from build123d import *
from build123d.topology import SkipClean

# Parameters (mm, degrees)
BOSS_EXTRUDE1_DEPTH       = 4
BOSS_EXTRUDE2_DEPTH       = 1
BOSS_EXTRUDE3_START       = -0.8
SKETCH4_R                 = 2
SKETCH4_R_2               = 1.25
BOSS_EXTRUDE3_DEPTH       = 3.2
MIRROR4_START             = -0.8
MIRROR4_COPY_1_SKETCH_R   = 2
MIRROR4_COPY_1_SKETCH_R_2 = 1.25
MIRROR4_COPY_1_DEPTH      = 3.2
SKETCH5_R                 = 4.5
CUT_EXTRUDE1_DEPTH        = 3
SKETCH1_R                 = 1.25
CUT_EXTRUDE2_DEPTH        = 10
FILLET2_R                 = 1
EXTRUDE_THIN1_START       = -4.2
SKETCH6_R                 = 2
SKETCH6_R_2               = 1
EXTRUDE_THIN1_DEPTH       = 4.2


with BuildPart() as part:
    # Sketch2 → Boss-Extrude1 (new body)
    with BuildSketch(Plane(origin=(0, 0, 0), x_dir=(1, 0, 0), z_dir=(0, 1, 0))):
        with BuildLine():
            Line((-26.6, 15.24), (-26.6, 2.54))
            ThreePointArc((-26.6, 2.54), (-25.504579362, -0.104579362), (-22.86, -1.2))
            Line((-22.86, -1.2), (-2.54, -1.2))
            ThreePointArc((-2.54, -1.2), (0.104579362, -0.104579362), (1.2, 2.54))
            Line((1.2, 2.54), (1.2, 15.24))
            ThreePointArc((1.2, 15.24), (0.104579362, 17.884579362), (-2.54, 18.98))
            Line((-2.54, 18.98), (-22.86, 18.98))
            ThreePointArc((-22.86, 18.98), (-25.504579362, 17.884579362), (-26.6, 15.24))
        make_face()
        with BuildLine():
            Line((0.2, 2.54), (0.2, 15.24))
            ThreePointArc((0.2, 15.24), (-0.60252742, 17.17747258), (-2.54, 17.98))
            Line((-2.54, 17.98), (-22.86, 17.98))
            ThreePointArc((-22.86, 17.98), (-24.79747258, 17.17747258), (-25.6, 15.24))
            Line((-25.6, 15.24), (-25.6, 2.54))
            ThreePointArc((-25.6, 2.54), (-24.79747258, 0.60252742), (-22.86, -0.2))
            Line((-22.86, -0.2), (-2.54, -0.2))
            ThreePointArc((-2.54, -0.2), (-0.60252742, 0.60252742), (0.2, 2.54))
        make_face(mode=Mode.SUBTRACT)
    extrude(amount=BOSS_EXTRUDE1_DEPTH)

    # Sketch3 → Boss-Extrude2 (add)
    with BuildSketch(Plane(origin=(0, 4, 0), x_dir=(1, 0, 0), z_dir=(0, 1, 0))):
        with BuildLine():
            Line((-26.6, 15.24), (-26.6, 2.54))
            ThreePointArc((-26.6, 2.54), (-25.504579362, -0.104579362), (-22.86, -1.2))
            Line((-22.86, -1.2), (-2.54, -1.2))
            ThreePointArc((-2.54, -1.2), (0.104579362, -0.104579362), (1.2, 2.54))
            Line((1.2, 2.54), (1.2, 15.24))
            ThreePointArc((1.2, 15.24), (0.104579362, 17.884579362), (-2.54, 18.98))
            Line((-2.54, 18.98), (-22.86, 18.98))
            ThreePointArc((-22.86, 18.98), (-25.504579362, 17.884579362), (-26.6, 15.24))
        make_face()
    extrude(amount=BOSS_EXTRUDE2_DEPTH)

    # Sketch4 → Boss-Extrude3 (add)
    # profile 1 of 2: a face of its own
    with BuildSketch(Plane.XZ.offset(BOSS_EXTRUDE3_START)):
        with BuildLine():
            ThreePointArc((-22.86, -4.54), (-24.274213562, -1.125786438), (-20.86, -2.54))
            Line((-20.86, -2.54), (-20.86, 0.2))
            Line((-20.86, 0.2), (-22.86, 0.2))
            ThreePointArc((-22.86, 0.2), (-24.79747258, -0.60252742), (-25.6, -2.54))
            Line((-25.6, -2.54), (-25.6, -4.54))
            Line((-25.6, -4.54), (-22.86, -4.54))
        make_face()
    # profile 2 of 2: a face of its own
    with BuildSketch(Plane.XZ.offset(BOSS_EXTRUDE3_START)):
        with Locations((-22.86, -2.54)):
            Circle(SKETCH4_R)
        with Locations(Location((-22.86, -2.54, 0), (0, 0, 90))):
            Circle(SKETCH4_R_2, mode=Mode.SUBTRACT)
    boss_extrude3 = extrude(amount=-BOSS_EXTRUDE3_DEPTH)

    # Mirror3: Boss-Extrude3 across plane
    add(boss_extrude3.mirror(Plane.ZY.offset(12.7)))

    # Mirror4: Boss-Extrude3 across plane
    add(boss_extrude3.mirror(Plane(origin=(0, 0, -8.89), x_dir=(1, 0, 0), z_dir=(0, 0, -1))))

    # Mirror4 copy 1 sketch → Mirror4 copy 1 (add)
    # profile 1 of 2: a face of its own
    with BuildSketch(Plane(origin=(-25.4, 0, -17.78), x_dir=(-1, 0, 0), z_dir=(0, -1, 0)).offset(MIRROR4_START)):
        with BuildLine():
            ThreePointArc((-22.86, -4.54), (-24.274213562, -1.125786438), (-20.86, -2.54))
            Line((-20.86, -2.54), (-20.86, 0.2))
            Line((-20.86, 0.2), (-22.86, 0.2))
            ThreePointArc((-22.86, 0.2), (-24.79747258, -0.60252742), (-25.6, -2.54))
            Line((-25.6, -2.54), (-25.6, -4.54))
            Line((-25.6, -4.54), (-22.86, -4.54))
        make_face()
    # profile 2 of 2: a face of its own
    with BuildSketch(Plane(origin=(-25.4, 0, -17.78), x_dir=(-1, 0, 0), z_dir=(0, -1, 0)).offset(MIRROR4_START)):
        with Locations((-22.86, -2.54)):
            Circle(MIRROR4_COPY_1_SKETCH_R)
        with Locations(Location((-22.86, -2.54, 0), (0, 0, 90))):
            Circle(MIRROR4_COPY_1_SKETCH_R_2, mode=Mode.SUBTRACT)
    extrude(amount=-MIRROR4_COPY_1_DEPTH)

    # Sketch5 → Cut-Extrude1 (cut)
    with BuildSketch(Plane(origin=(0, 5, 0), x_dir=(1, 0, 0), z_dir=(0, 1, 0))):
        with Locations(Location((-12.7, 8.89, 0), (0, 0, 270))):
            Circle(SKETCH5_R)
    extrude(amount=-CUT_EXTRUDE1_DEPTH, mode=Mode.SUBTRACT)

    # Sketch1 → Cut-Extrude2 (cut)
    with SkipClean():  # the faces are left unmerged after this step: merging them gives an invalid solid
        with BuildSketch(Plane(origin=(0, 0, 0), x_dir=(1, 0, 0), z_dir=(0, 1, 0))):
            with Locations(Location((-22.86, 2.54, 0), (0, 0, 270))):
                Circle(SKETCH1_R)
            with Locations(Location((-2.54, 2.54, 0), (0, 0, 270))):
                Circle(SKETCH1_R)
            with Locations(Location((-2.54, 15.24, 0), (0, 0, 270))):
                Circle(SKETCH1_R)
            with Locations(Location((-22.86, 15.24, 0), (0, 0, 270))):
                Circle(SKETCH1_R)
        extrude(amount=CUT_EXTRUDE2_DEPTH, mode=Mode.SUBTRACT)
    add(part.part.scale(1), mode=Mode.REPLACE)  # the faces are merged on a copy

    # Fillet2
    fillet2_edges = [part.edges().sort_by_distance(p)[0] for p in [
        (-4.54, 2.4, 0.2),
        (0.2, 2.4, -4.54),
        (0.2, 2.4, -13.24),
        (-4.54, 2.4, -17.98),
        (-20.86, 2.4, -17.98),
        (-25.6, 2.4, -13.24),
        (-25.6, 2.4, -4.54),
        (-20.86, 2.4, 0.2),
    ]]
    fillet(fillet2_edges, radius=FILLET2_R)

    # Sketch6 → Extrude-Thin1 (add)
    # profile 1 of 4: a face of its own
    with BuildSketch(Plane(origin=(0, 5, 0), x_dir=(1, 0, 0), z_dir=(0, 1, 0)).offset(EXTRUDE_THIN1_START)):
        with Locations((-2.54, 15.24)):
            Circle(SKETCH6_R)
        with Locations((-2.54, 15.24)):
            Circle(SKETCH6_R_2, mode=Mode.SUBTRACT)
    # profile 2 of 4: a face of its own
    with BuildSketch(Plane(origin=(0, 5, 0), x_dir=(1, 0, 0), z_dir=(0, 1, 0)).offset(EXTRUDE_THIN1_START)):
        with Locations((-22.86, 15.24)):
            Circle(SKETCH6_R)
        with Locations((-22.86, 15.24)):
            Circle(SKETCH6_R_2, mode=Mode.SUBTRACT)
    # profile 3 of 4: a face of its own
    with BuildSketch(Plane(origin=(0, 5, 0), x_dir=(1, 0, 0), z_dir=(0, 1, 0)).offset(EXTRUDE_THIN1_START)):
        with Locations((-2.54, 2.54)):
            Circle(SKETCH6_R)
        with Locations((-2.54, 2.54)):
            Circle(SKETCH6_R_2, mode=Mode.SUBTRACT)
    # profile 4 of 4: a face of its own
    with BuildSketch(Plane(origin=(0, 5, 0), x_dir=(1, 0, 0), z_dir=(0, 1, 0)).offset(EXTRUDE_THIN1_START)):
        with Locations((-22.86, 2.54)):
            Circle(SKETCH6_R)
        with Locations((-22.86, 2.54)):
            Circle(SKETCH6_R_2, mode=Mode.SUBTRACT)
    extrude(amount=EXTRUDE_THIN1_DEPTH)


solid = part.part
Geometry check sheet. Reference: the model listing, model coordinates, mm. A direction names the side the tool comes from. Coordinates: 2 decimals unless noted, no trailing zeros. Order: outer loops, then holes, each group sorted by start corner. A loop starts at its lowest first (then second) coordinate and runs counter-clockwise, first axis right, second up. Notation, with made-up numbers: (-29, 60) - (2, 60) arc R4 ccw to (2, 64) - close; hole circle Ø7 at (-15, 83.25). An arc over 180 degrees is marked (long way). One line per item, written item: value.
(1) Thickness scan on probe 1 along X at (y, z) = (3.3, -15.24); probe 2 along Z at (x, y) = (-22.86, 2.7); probe 3 along Z at (x, y) = (-8.75, 2.15). Record the ranges inside material, lowest first. Write a range as from..to.
Data:
probe 1: x = -26.6..-23.86, -21.86..-20.86, -4.54..-3.54, -1.54..1.2
probe 2: z = -18.98..-16.24, -14.24..-13.24, -4.54..-3.54, -1.54..1.2
probe 3: z = -18.98..-17.98, 0.2..1.2
(2) Sectioned sample at D-D (z = -15.75). Enter the section's corners in (x, y), and give its area (3 significant figures).
Data:
outline: (-26.57, 0) - (-25.55, 0) - (-25.55, 0.8) - (-23.72, 0.8) - (-23.72, 5) - (-26.57, 5) - close; (-22, 0.8) - (-20.86, 0.8) - (-20.86, 4) - (-4.54, 4) - (-4.54, 0.8) - (-3.4, 0.8) - (-3.4, 5) - (-22, 5) - close; (-1.68, 0.8) - (0.15, 0.8) - (0.15, 0) - (1.17, 0) - (1.17, 5) - (-1.68, 5) - close
area: 51.4 mm^2
(3) Depth check by flat-ended pin: pin 1 Ø0.5 at (x, y) = (-23.5, 2.5) entering from +Z; pin 2 Ø3 at (x, z) = (-3, -2.5) entering from -Y; pin 3 Ø1.2 at (x, z) = (-22.86, -15.24) entering from -Y. Enter the tip coordinate at first touch or a pass-through.
Data:
pin 1: stops at z = 1.18
pin 2: stops at y = 0.8
pin 3: passes through
(4) Sectioned sample at A-A (z = -8.89). Enter the section's corners in (x, y).
Data:
outline: (-26.6, 0) - (-25.6, 0) - (-25.6, 4) - (-17.2, 4) - (-17.2, 5) - (-26.6, 5) - close; (-8.2, 4) - (0.2, 4) - (0.2, 0) - (1.2, 0) - (1.2, 5) - (-8.2, 5) - close
(5) Sectioned sample at B-B (x = -12.7). Enter the section's corners in (y, z).
Data:
outline: (0, -18.98) - (5, -18.98) - (5, -13.39) - (4, -13.39) - (4, -17.98) - (0, -17.98) - close; (0, 0.2) - (4, 0.2) - (4, -4.39) - (5, -4.39) - (5, 1.2) - (0, 1.2) - close
(6) Access from +Z, -Z, +X, -X, +Y, -Y to the whole of each face (thin tool, end or side, straight path). Record for faces 5 (the face through (0.2, 2, -9)), 6 (the face through (0.13, 2.46, -17.86)).
Data:
face 5: -Y
face 6: -Z, +X, +Y, -Y
(7) Sectioned sample at C-C (y = 4.6). Enter the section's corners in (x, z), and give its area (3 significant figures).
Data:
outline: (-26.6, -15.24) arc R3.74 ccw to (-22.86, -18.98) - (-2.54, -18.98) arc R3.74 ccw to (1.2, -15.24) - (1.2, -2.54) arc R3.74 ccw to (-2.54, 1.2) - (-22.86, 1.2) arc R3.74 ccw to (-26.6, -2.54) - close; hole circle Ø2 at (-22.86, -15.24); hole circle Ø2 at (-22.86, -2.54); hole circle Ø9 at (-12.7, -8.89); hole circle Ø2 at (-2.54, -15.24); hole circle Ø2 at (-2.54, -2.54)
area: 473 mm^2
(8) Release check for a two-part mould opening along X. For faces 1 (the face through (-2, 2, -4.54)), 2 (the face through (-20.559, 2.422, -17.695)), 3 (the face through (-13, 2, -18.98)), 4 (the face through (1.2, 2, -9)) record: +X half, -X half, draft (parallel to the pull), parting line (faces both ways), or undercut.
Data:
face 1: undercut
face 2: undercut
face 3: draft
face 4: +X half
